```python
from build123d import *

# Parameters (mm, degrees)
F0_R     = 12.7
F1_DEPTH = 25.4


with BuildPart() as f1:
    # F0 (on Top) → F1 (new body)
    with BuildSketch(Plane.XY):
        with BuildLine():
            Line((-457.2, -914.4), (457.2, -914.4))
            Line((457.2, -914.4), (457.2, -635))
            ThreePointArc((457.2, -635), (431.8, -609.6), (457.2, -584.2))
            Line((457.2, -584.2), (457.2, -330.2))
            ThreePointArc((457.2, -330.2), (431.8, -304.8), (457.2, -279.4))
            Line((457.2, -279.4), (457.2, -25.4))
            ThreePointArc((457.2, -25.4), (431.8, 0), (457.2, 25.4))
            Line((457.2, 25.4), (457.2, 279.4))
            ThreePointArc((457.2, 279.4), (431.8, 304.8), (457.2, 330.2))
            Line((457.2, 330.2), (457.2, 584.2))
            ThreePointArc((457.2, 584.2), (431.8, 609.6), (457.2, 635))
            Line((457.2, 635), (457.2, 914.4))
            Line((457.2, 914.4), (-457.2, 914.4))
            Line((-457.2, 914.4), (-457.2, 635))
            ThreePointArc((-457.2, 635), (-431.8, 609.6), (-457.2, 584.2))
            Line((-457.2, 584.2), (-457.2, 330.2))
            ThreePointArc((-457.2, 330.2), (-431.8, 304.8), (-457.2, 279.4))
            Line((-457.2, 279.4), (-457.2, 25.4))
            ThreePointArc((-457.2, 25.4), (-431.8, 0), (-457.2, -25.4))
            Line((-457.2, -25.4), (-457.2, -279.4))
            ThreePointArc((-457.2, -279.4), (-431.8, -304.8), (-457.2, -330.2))
            Line((-457.2, -330.2), (-457.2, -584.2))
            ThreePointArc((-457.2, -584.2), (-431.8, -609.6), (-457.2, -635))
            Line((-457.2, -635), (-457.2, -914.4))
        make_face()
        with Locations((-406.4, -762)):
            Circle(F0_R, mode=Mode.SUBTRACT)
        with Locations((-431.8, -457.2)):
            Circle(F0_R, mode=Mode.SUBTRACT)
        with Locations((-406.4, -152.4)):
            Circle(F0_R, mode=Mode.SUBTRACT)
        with Locations((406.4, -762)):
            Circle(F0_R, mode=Mode.SUBTRACT)
        with Locations((406.4, -457.2)):
            Circle(F0_R, mode=Mode.SUBTRACT)
        with Locations((406.4, -152.4)):
            Circle(F0_R, mode=Mode.SUBTRACT)
        with Locations((-406.4, 152.4)):
            Circle(F0_R, mode=Mode.SUBTRACT)
        with Locations((-419.1, 457.2)):
            Circle(F0_R, mode=Mode.SUBTRACT)
        with Locations((-431.8, 762)):
            Circle(F0_R, mode=Mode.SUBTRACT)
        with Locations((406.4, 152.4)):
            Circle(F0_R, mode=Mode.SUBTRACT)
        with Locations((406.4, 457.2)):
            Circle(F0_R, mode=Mode.SUBTRACT)
        with Locations((406.4, 762)):
            Circle(F0_R, mode=Mode.SUBTRACT)
    extrude(amount=F1_DEPTH)


solid = f1.part
```
Design review of the part built by this model. Coordinates are the model's own, in mm. Round coordinates to 2 decimals unless told otherwise and drop trailing zeros. Write each loop counter-clockwise with the first axis right and the second up, starting at its lowest first coordinate (ties: lowest second). Pieces come first, ordered by that corner, then holes.
Item 1: We need section A-A on y = 304.8. Write out the cut boundary in (x, z), and give its area (3 significant figures).
Item 2: Clearance check with a flat-ended pin moving along its axis: pin 1 Ø20.5 at (x, y) = (406.4, -457.2) entering from -Z. State where the tip first meets the part, or that it passes through.
Item 3: For probe 1 along X at (y, z) = (-762, 13.5); probe 2 along X at (y, z) = (-463, 9.5); probe 3 along X at (y, z) = (16.5, 18.75), list the stretches that pass through material, from the lowest coordinate up.
Returned:
1. outline: (-431.8, 0) - (431.8, 0) - (431.8, 25.4) - (-431.8, 25.4) - close
1. area: 21,900 mm2
2. pin 1: passes through
3. probe 1: x = -457.2 to -419.1, -393.7 to 393.7, 419.1 to 457.2
3. probe 2: x = -457.2 to -443.1, -420.5 to 395.1, 417.7 to 457.2
3. probe 3: x = -437.89 to 437.89
